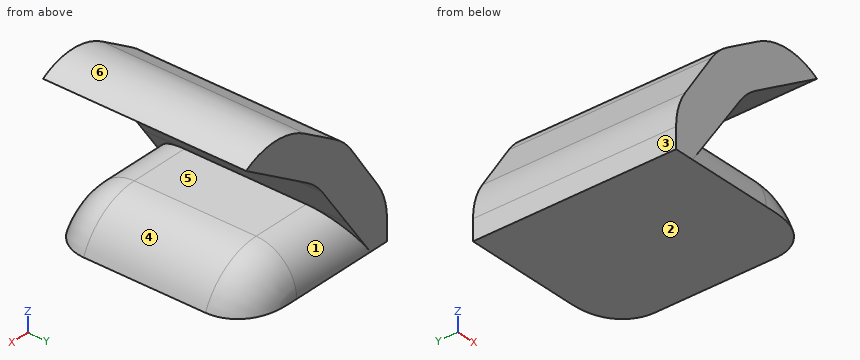
```python
from build123d import *

# Parameters (mm, degrees)
F1_DEPTH     = 12.5
F2_T1_DEPTH  = 75.8666564448
F2_T3_DEPTH  = 33.4238697913
F2_T5_DEPTH  = 37.1110249992
F2_T7_DEPTH  = 61.9747717196
F3_T2_ANGLE  = 157.1183672373
F3_T4_ANGLE  = 157.1183672373
F3_T8_DEPTH  = 19.8096921988
F3_T13_DEPTH = 19.8096921988
F4_R         = 8


# Not quite as in the source:
# - a fillet or chamfer that OpenCascade refuses, or shapes differently, is made with other operations: its cross-section is extruded or revolved along the edge and cut away or added


with BuildPart() as f1:
    # F0 (on Front) → F1 (new body, symmetric)
    with BuildSketch(Plane.XZ):
        Polygon((-20.558629185, 0), (0, 0), (0, 4.9480088055), (-14.7046465427, 4.9480088055), (-10.2444691584, 11.3595137373), (0, 17.8922185832), (0, 23.3462397009), (-14.4258858636, 14.1471242532), (-20.558629185, 4.9480088055), align=None)
    extrude(amount=F1_DEPTH, both=True)

    # F2: fillet of radius 8 on 4 edges, made by hand

    # F2_s2 → F2_t1 (cut)
    with BuildSketch(Plane.XZ.offset(-37.9333282224)):
        with BuildLine():
            ThreePointArc((-8.5777252412, 17.8763860282), (-4.2911639454, 19.1311087323), (0, 17.8922185832))
            Line((0, 17.8922185832), (0, 23.3462397009))
            Line((0, 23.3462397009), (-8.5777252412, 17.8763860282))
        make_face()
    extrude(amount=F2_T1_DEPTH, mode=Mode.SUBTRACT)

    # F2_s4 → F2_t3 (cut)
    with BuildSketch(Plane.XZ.offset(-16.7119348957)):
        with BuildLine():
            ThreePointArc((-15.3604302761, 12.7453075635), (-14.3030712709, 14.0217863385), (-13.0053552923, 15.0529698176))
            Line((-13.0053552923, 15.0529698176), (-14.4258858636, 14.1471242532))
            Line((-14.4258858636, 14.1471242532), (-15.3604302761, 12.7453075635))
        make_face()
    extrude(amount=F2_T3_DEPTH, mode=Mode.SUBTRACT)

    # F2_s6 → F2_t5 (cut)
    with BuildSketch(Plane.XZ.offset(-18.5555124996)):
        with BuildLine():
            ThreePointArc((-20.558629185, 2.5258038057), (-20.215365424, 4.8440769057), (-19.2150316433, 6.96340522))
            Line((-19.2150316433, 6.96340522), (-20.558629185, 4.9480088055))
            Line((-20.558629185, 4.9480088055), (-20.558629185, 2.5258038057))
        make_face()
    extrude(amount=F2_T5_DEPTH, mode=Mode.SUBTRACT)

    # F2_s8 → F2_t7 (cut)
    with BuildSketch(Plane.XZ.offset(-30.9873858598)):
        with BuildLine():
            ThreePointArc((-7.3949543439, 4.9480088055), (-2.9461303171, 3.5969158419), (0, 0))
            Line((0, 0), (0, 4.9480088055))
            Line((0, 4.9480088055), (-7.3949543439, 4.9480088055))
        make_face()
    extrude(amount=F2_T7_DEPTH, mode=Mode.SUBTRACT)

    # F3: fillet of radius 5 on 4 edges, made by hand

    # F3_s1 → F3_t2 (revolve, cut)
    with BuildSketch(Plane.YZ.offset(-7.3949543439)):
        with BuildLine():
            ThreePointArc((12.5, -0.0519911945), (11.0355339059, 3.4835427114), (7.5, 4.9480088055))
            Line((7.5, 4.9480088055), (12.5, 4.9480088055))
            Line((12.5, 4.9480088055), (12.5, -0.0519911945))
        make_face()
    revolve(axis=Axis((-7.3949543439, 12.5, -3.0519911944), (0, 1, 0)), revolution_arc=F3_T2_ANGLE, mode=Mode.SUBTRACT)

    # F3_s3 → F3_t4 (revolve, cut)
    with BuildSketch(Plane.YZ.offset(-7.3949543439)):
        with BuildLine():
            ThreePointArc((-12.5, -0.0519911945), (-11.0355339059, 3.4835427114), (-7.5, 4.9480088055))
            Line((-7.5, 4.9480088055), (-12.5, 4.9480088055))
            Line((-12.5, 4.9480088055), (-12.5, -0.0519911945))
        make_face()
    revolve(axis=Axis((-7.3949543439, -12.5, -3.0519911944), (0, 1, 0)), revolution_arc=F3_T4_ANGLE, mode=Mode.SUBTRACT)


with BuildPart() as f3_tool6:
    # F3_s7 → F3_t8 (new body)
    with BuildSketch(Plane.YZ.offset(-7.3949543439)):
        with BuildLine():
            ThreePointArc((-12.5, -0.0519911945), (-11.0355339059, 3.4835427114), (-7.5, 4.9480088055))
            Line((-7.5, 4.9480088055), (-12.5, 4.9480088055))
            Line((-12.5, 4.9480088055), (-12.5, -0.0519911945))
        make_face()
    extrude(amount=-F3_T8_DEPTH)

    split(bisect_by=Plane(origin=(-12.2288219378, 0, 8.5070066427), x_dir=(0, 1, 0), z_dir=(0.8209051994, 0, -0.5710644917)), keep=Keep.TOP)


with BuildPart() as f1_1:
    add(f1.part)

    # F3_t5: cut F3_tool6
    add(f3_tool6.part, mode=Mode.SUBTRACT)


with BuildPart() as f3_tool11:
    # F3_s12 → F3_t13 (new body)
    with BuildSketch(Plane.YZ.offset(-7.3949543439)):
        with BuildLine():
            ThreePointArc((12.5, -0.0519911945), (11.0355339059, 3.4835427114), (7.5, 4.9480088055))
            Line((7.5, 4.9480088055), (12.5, 4.9480088055))
            Line((12.5, 4.9480088055), (12.5, -0.0519911945))
        make_face()
    extrude(amount=-F3_T13_DEPTH)

    split(bisect_by=Plane(origin=(-12.2288219378, 0, 8.5070066427), x_dir=(0, 1, 0), z_dir=(0.8209051994, 0, -0.5710644917)), keep=Keep.TOP)


with BuildPart() as f1_2:
    add(f1_1.part)

    # F3_t10: cut F3_tool11
    add(f3_tool11.part, mode=Mode.SUBTRACT)

    # F4
    f4_edges = [f1_2.edges().sort_by_distance(p)[0] for p in [
        (-10.244469, 0, 11.359514),
    ]]
    fillet(f4_edges, radius=F4_R)


solid = f1_2.part
```
The listing builds one solid part. Answer for the finished solid, in the listing's coordinates (mm). Face numbers are marked on the shaded views. A direction names the side the tool comes from. Coordinates: 2 decimals unless noted, no trailing zeros. Loops run counter-clockwise (first coordinate to the right, second up) from the corner with the lowest first, then second, coordinate; pieces in that order, holes last. Notation, with made-up numbers: (19.5, 37) - (74.5, 37) arc R13 cw to (74.5, 50) - close; hole circle Ø11 at (-33.5, 2). An arc over 180 degrees is marked (long way). Use a Markdown table: item, result. Add a question column.
1) For the marked faces 1 and 2, determine the directions among +Z, -Z, +X, -X, +Y, -Y from which every point of the face is accessible in a straight line to the end or side of a thin tool.
2) The part is cut by section B-B, the plane x = -14.25. Give the vertices of the cut face in (y, z), and give its area (3 significant figures).
3) Find the intervals of material crossed by line 1 (Z direction, x = -4.75, y = 5.5); line 2 (Z direction, x = -13, y = -1.5); line 3 (X direction, y = 5, z = 15.75), in increasing order.
4) The mould has two halves that part along Z. Classify the marked faces 3, 4, 5 and 6: released by +Z, released by -Z, zero draft, split by the parting line, or undercut.
5) The part is cut by section A-A, the plane y = 0.25. Give the vertices of the cut face in (x, z).
6) The part is cut by section C-C, the plane z = 10.75. Give the vertices of the cut face in (x, y), and give its area (3 significant figures).
7) Given pin 1 (1 mm diameter, centred on y = -1.5, z = 14, fed in from +X); pin 2 (2 mm diameter, centred on x = -11, y = 3, fed in from +Z); pin 3 (4 mm diameter, centred on y = 5.5, z = 12.5, fed in from -X); pin 4 (2 mm diameter, centred on x = -5.5, z = 6.5, fed in from +Y), each flat-ended and moving along its own axis, determine where each tip first touches the part or whether it passes through.
8) The part is cut by section D-D, the plane z = 16. Give the vertices of the cut face in (x, y), and give its area (3 significant figures).
Here are the results:
| question | item | result |
|---|---|---|
| 1 | face 1 | +X, +Y |
| 1 | face 2 | -Z, +X, -X, +Y, -Y |
| 2 | outline | (-12.5, 0) - (12.5, 0) arc R5 ccw to (7.5, 4.95) - (-7.5, 4.95) arc R5 ccw to start; (-12.5, 5.6) - (12.5, 5.6) - (12.5, 14.07) - (-12.5, 14.07) - close |
| 2 | area | 325 mm^2 |
| 3 | line 1 | z = 0 to 4.5, 14.86 to 19.12 |
| 3 | line 2 | z = 0 to 4.95, 7.4 to 15.06 |
| 3 | line 3 | x = -11.91 to -3.36 |
| 4 | face 3 | zero draft |
| 4 | face 4 | undercut |
| 4 | face 5 | undercut |
| 4 | face 6 | released by +Z |
| 5 | outline | (-20.56, 0) - (0, 0) arc R8 ccw to (-7.39, 4.95) - (-14.7, 4.95) - (-11.16, 10.04) arc R8 cw to (-8.89, 12.22) - (0, 17.89) arc R8 ccw to (-8.58, 17.88) - (-13.01, 15.05) arc R8 ccw to (-15.36, 12.75) - (-19.22, 6.96) arc R8 ccw to (-20.56, 2.53) - close |
| 6 | outline | (-16.69, -12.5) - (-10.61, -12.5) - (-10.61, 12.5) - (-16.69, 12.5) - close |
| 6 | area | 152 mm^2 |
| 7 | pin 1 | stops at x = -5.32 |
| 7 | pin 2 | stops at z = 16.97 |
| 7 | pin 3 | stops at x = -16.86 |
| 7 | pin 4 | passes through |
| 8 | outline | (-11.52, -12.5) - (-2.97, -12.5) - (-2.97, 12.5) - (-11.52, 12.5) - close |
| 8 | area | 214 mm^2 |
